For this review, take the finished solid that the model builds, in its own axes (mm). A direction names the side the tool comes from. Coordinates: 2 decimals unless noted, no trailing zeros. Loops run counter-clockwise (first coordinate to the right, second up) from the corner with the lowest first, then second, coordinate; pieces in that order, holes last. Notation, with made-up numbers: M 6.5,-13 L 62.5,-13 A23 cw 62.5,-2 Z; hole C 9,8.25 d11. An arc over 180 degrees is marked long. Put each result on its own line as item: value.
```python
from build123d import *

# Parameters (mm, degrees)
SKETCH1_W           = 95
SKETCH1_H           = 65
BOSS_EXTRUDE1_DEPTH = 30
FILLET1_R           = 5
SKETCH2_W           = 75
SKETCH2_H           = 50
CUT_EXTRUDE1_DEPTH  = 25
SKETCH3_R           = 1.5
BOSS_EXTRUDE2_DEPTH = 5
SKETCH4_W           = 45
SKETCH4_H           = 40
CUT_EXTRUDE2_DEPTH  = 107.330851591
SKETCH5_W           = 70
SKETCH5_H           = 40
CUT_EXTRUDE3_DEPTH  = 88.78524933


with BuildPart() as part:
    # Sketch1 → Boss-Extrude1 (new body)
    with BuildSketch(Plane(origin=(0, 0, 0), x_dir=(1, 0, 0), z_dir=(0, 1, 0))):
        Rectangle(SKETCH1_W, SKETCH1_H)
    extrude(amount=BOSS_EXTRUDE1_DEPTH)

    # Fillet1
    fillet1_edges = [part.edges().sort_by_distance(p)[0] for p in [
        (47.5, 15, 32.5),
        (-47.5, 15, 32.5),
        (-47.5, 15, -32.5),
        (47.5, 15, -32.5),
    ]]
    fillet(fillet1_edges, radius=FILLET1_R)

    # Sketch2 → Cut-Extrude1 (cut)
    with BuildSketch(Plane(origin=(0, 30, 0), x_dir=(1, 0, 0), z_dir=(0, 1, 0))):
        Rectangle(SKETCH2_W, SKETCH2_H)
    extrude(amount=-CUT_EXTRUDE1_DEPTH, mode=Mode.SUBTRACT)

    # Sketch3 → Boss-Extrude2 (add)
    with BuildSketch(Plane(origin=(0, 30, 0), x_dir=(1, 0, 0), z_dir=(0, 1, 0))):
        with Locations(Location((43, 28, 0), (0, 0, 270))):
            Circle(SKETCH3_R)
        with Locations(Location((-43, 28, 0), (0, 0, 270))):
            Circle(SKETCH3_R)
        with Locations(Location((43, -28, 0), (0, 0, 270))):
            Circle(SKETCH3_R)
        with Locations(Location((-43, -28, 0), (0, 0, 270))):
            Circle(SKETCH3_R)
    extrude(amount=BOSS_EXTRUDE2_DEPTH)

    # Sketch4 → Cut-Extrude2 (cut, through all)
    with BuildSketch(Plane(origin=(47.5, 0, 0), x_dir=(0, 0, -1), z_dir=(1, 0, 0))):
        with Locations((0, 30)):
            Rectangle(SKETCH4_W, SKETCH4_H)
    extrude(amount=-CUT_EXTRUDE2_DEPTH, mode=Mode.SUBTRACT)

    # Sketch5 → Cut-Extrude3 (cut, through all)
    with BuildSketch(Plane.XY.offset(32.5)):
        with Locations((0, 30)):
            Rectangle(SKETCH5_W, SKETCH5_H)
    extrude(amount=-CUT_EXTRUDE3_DEPTH, mode=Mode.SUBTRACT)


solid = part.part
```
(1) Add section C-C (y = 7.5). Write out the cut boundary in (x, z), plus the area to 3 significant figures.
Determined:
outline: M -47.5,-27.5 A5 ccw -42.5,-32.5 L 42.5,-32.5 A5 ccw 47.5,-27.5 L 47.5,27.5 A5 ccw 42.5,32.5 L -42.5,32.5 A5 ccw -47.5,27.5 Z; hole M -37.5,-25 L 37.5,-25 L 37.5,25 L -37.5,25 Z
area: 2,400 mm^2
(2) For pin 1 (6 mm diameter, centred on x = -14, z = 27, fed in from +Y); pin 2 (4 mm diameter, centred on x = 27.5, z = -22, fed in from +Y), all flat-tipped, find the tip position at first contact; note any pin that passes through.
Determined:
pin 1: stops at y = 10
pin 2: stops at y = 5
(3) Draft analysis for pull direction Z (two halves, no side actions). For faces 1 (the flat face through (-1, 0, 0)), 2 (the cylindrical face through (-43.9, 32.5, -29.2)), 3 (the cylindrical face through (46.07, 15.21, -31)), state which applies: +Z half, -Z half, draft (parallel to the pull), parting line (faces both ways), or undercut.
Determined:
face 1: draft
face 2: undercut
face 3: -Z half
(4) Tool access review of faces 4 (the flat face through (-42, 10, 0)), 5 (the cylindrical face through (41.536, 32.465, -28.325)), 6 (the flat face through (-35, 20, -29)): name each direction out of +Z, -Z, +X, -X, +Y, -Y from which nothing blocks a thin tool from reaching the whole face with its end or side.
Determined:
face 4: +X, -X, +Y
face 5: +Y
face 6: +Z, -Z, +Y
(5) Add section D-D (x = -11). Write out the cut boundary in (y, z), plus the area to 3 significant figures.
Determined:
outline: M 0,-32.5 L 10,-32.5 L 10,-25 L 5,-25 L 5,25 L 10,25 L 10,32.5 L 0,32.5 Z
area: 400 mm^2
(6) Add section A-A (y = 23.5). Write out the cut boundary in (x, z).
Determined:
outline: M -47.5,-27.5 A5 ccw -42.5,-32.5 L -35,-32.5 L -35,-25 L -37.5,-25 L -37.5,-22.5 L -47.5,-22.5 Z; M -47.5,22.5 L -37.5,22.5 L -37.5,25 L -35,25 L -35,32.5 L -42.5,32.5 A5 ccw -47.5,27.5 Z; M 35,-32.5 L 42.5,-32.5 A5 ccw 47.5,-27.5 L 47.5,-22.5 L 37.5,-22.5 L 37.5,-25 L 35,-25 Z; M 35,25 L 37.5,25 L 37.5,22.5 L 47.5,22.5 L 47.5,27.5 A5 ccw 42.5,32.5 L 35,32.5 Z
(7) Wall thickness on line 1 along X through (y, z) = (8, 0); line 2 along Z through (x, y) = (23, 8); line 3 along X through (y, z) = (14.5, 27.5): over which ranges is each line inside the solid? List them lowest first. Write a range as [from, to].
Determined:
line 1: x = [-47.5, -37.5], [37.5, 47.5]
line 2: z = [-32.5, -25], [25, 32.5]
line 3: x = [-47.5, -35], [35, 47.5]
(8) Add section B-B (z = -5). Write out the cut boundary in (x, y).
Determined:
outline: M -47.5,0 L 47.5,0 L 47.5,10 L 37.5,10 L 37.5,5 L -37.5,5 L -37.5,10 L -47.5,10 Z
